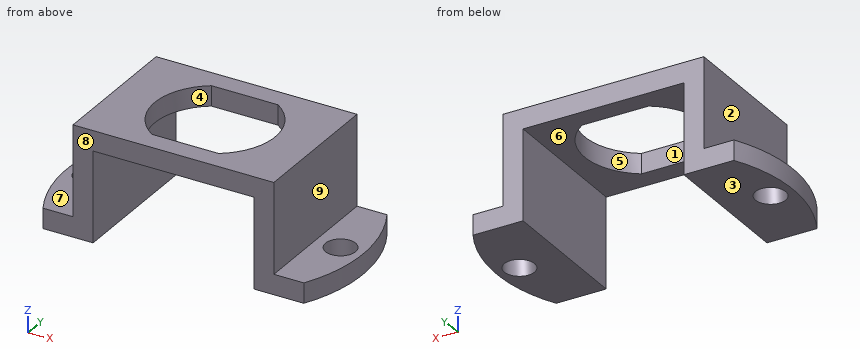
from build123d import *

# Parameters (mm, degrees)
BOSS_EXTRUDE1_DEPTH = 14
SKETCH3_R           = 1.5
CUT_EXTRUDE1_DEPTH  = 14
CUT_EXTRUDE2_START  = -2
CUT_EXTRUDE2_DEPTH  = 2


# Read off the part's stored shape, not the designer's step: Cut-Extrude2
with BuildPart() as part:
    # Sketch2 → Boss-Extrude1 (new body)
    with BuildSketch(Plane(origin=(0, 0, 0), x_dir=(1, 0, 0), z_dir=(0, 1, 0))):
        Polygon((-10, 0), (10, 0), (10, 9), (15, 9), (15, 11), (8, 11), (8, 2), (-8, 2), (-8, 11), (-15, 11), (-15, 9), (-10, 9), align=None)
    extrude(amount=BOSS_EXTRUDE1_DEPTH)

    # Sketch3 → Cut-Extrude1 (cut)
    with BuildSketch(Plane.XY):
        with Locations((-12.5, 7)):
            Circle(SKETCH3_R)
        with Locations((12.5, 7)):
            Circle(SKETCH3_R)
        with BuildLine():
            Line((-3.31662479, 2), (3.31662479, 2))
            ThreePointArc((3.31662479, 2), (6, 7), (3.31662479, 12))
            Line((3.31662479, 12), (-3.31662479, 12))
            ThreePointArc((-3.31662479, 12), (-6, 7), (-3.31662479, 2))
        make_face()
    extrude(amount=-CUT_EXTRUDE1_DEPTH, mode=Mode.SUBTRACT)

    # Cut-Extrude2 outline → Cut-Extrude2 (cut)
    with BuildSketch(Plane.XY.offset(-9).offset(CUT_EXTRUDE2_START)):
        with BuildLine():
            ThreePointArc((-12.983162173, 0), (-14.75, 7), (-12.983162173, 14))
            Line((-12.983162173, 14), (-15, 14))
            Line((-15, 14), (-15, 0))
            Line((-15, 0), (-12.983162173, 0))
        make_face()
        with BuildLine():
            Line((15, 14), (12.983162173, 14))
            ThreePointArc((12.983162173, 14), (14.75, 7), (12.983162173, 0))
            Line((12.983162173, 0), (15, 0))
            Line((15, 0), (15, 14))
        make_face()
    extrude(amount=CUT_EXTRUDE2_DEPTH, mode=Mode.SUBTRACT)


solid = part.part
Design review of the part built by this model. Coordinates are the model's own, in mm. Face numbers are marked on the shaded views. A direction names the side the tool comes from. Give positions to 0.01 mm unless a question says otherwise; leave off trailing zeros. Loops run counter-clockwise (first coordinate to the right, second up) from the corner with the lowest first, then second, coordinate; pieces in that order, holes last. Notation, with made-up numbers: (50, 22) -> (96, 22) arc R32 cw to (96, 48) -> close; hole circle Ø5 at (-33.75, -30.5). An arc over 180 degrees is marked (long way). One line per question, with ' | ' between items. Start each with the question number.
(1) We need section A-A (y = 7). State the section outline as (x, z) points, and give its area (3 significant figures).
(2) We need section D-D (z = -1). State the section outline as (x, y) points, and give its area (3 significant figures).
(3) Draft analysis for pull direction X (two halves, no side actions). For the marked faces 1, 2, 3 and 4, state which applies: +X half, -X half, draft (parallel to the pull), parting line (faces both ways), or undercut.
(4) For the marked faces 5, 6, 7, 8 and 9, list the 3-axis set-ups (+Z, -Z, +X, -X, +Y, -Y) from which the entire face can be reached by the end or side of a thin tool; tool diameter is ignored.
(5) For line 1 (Y direction, x = -12.5, z = -10.3); line 2 (Y direction, x = -0.25, z = -1.25); line 3 (X direction, y = 6.25, z = -7), list the stretches that pass through material, from the lowest coordinate up.
(6) We need section B-B (z = -5.25). State the section outline as (x, y) points.
(7) We need section C-C (x = 12.5). State the section outline as (y, z) points, and give its area (3 significant figures).
(8) Insertion check: P1, Ø2, axis at y = 3.5, z = -2.5, coming from the +X side; P2, Ø4, axis at x = -4.5, z = -5.5, coming from the +Y side; P3, Ø6, axis at y = 4, z = -3.5, coming from the -X side; P4, Ø2.5, axis at y = 9.5, z = -8, coming from the +X side. Each pin has a flat end and moves straight along its axis. Give the tip position at first contact, or say it passes through.
The answers:
1) outline: (-14.75, -11) -> (-14, -11) -> (-14, -9) -> (-14.75, -9) -> close; (-11, -11) -> (-8, -11) -> (-8, -2) -> (-6, -2) -> (-6, 0) -> (-10, 0) -> (-10, -9) -> (-11, -9) -> close; (6, -2) -> (8, -2) -> (8, -11) -> (11, -11) -> (11, -9) -> (10, -9) -> (10, 0) -> (6, 0) -> close; (14, -11) -> (14.75, -11) -> (14.75, -9) -> (14, -9) -> close | area: 59.0 mm^2
2) outline: (-10, 0) -> (10, 0) -> (10, 14) -> (-10, 14) -> close; hole (-3.32, 2) -> (3.32, 2) arc R6 ccw to (3.32, 12) -> (-3.32, 12) arc R6 ccw to start | area: 176 mm^2
3) face 1: undercut | face 2: -X half | face 3: draft | face 4: undercut
4) face 5: +Z, -Z | face 6: -Z, +Y, -Y | face 7: +Z, -X, +Y, -Y | face 8: +Z, -Z, +X, -X, -Y | face 9: +Z, +X, +Y, -Y
5) line 1: y = 0 to 5.5, 8.5 to 14 | line 2: y = 0 to 2, 12 to 14 | line 3: x = -10 to -8, 8 to 10
6) outline: (-10, 0) -> (-8, 0) -> (-8, 14) -> (-10, 14) -> close; (8, 0) -> (10, 0) -> (10, 14) -> (8, 14) -> close
7) outline: (0, -11) -> (5.5, -11) -> (5.5, -9) -> (0, -9) -> close; (8.5, -11) -> (14, -11) -> (14, -9) -> (8.5, -9) -> close | area: 22.0 mm^2
8) P1: stops at x = 10 | P2: passes through | P3: stops at x = -10 | P4: stops at x = 14.65
